Autodesk Inventor part; units mm, degrees
ref_plane "YZ Plane" through (0, 0, 0) normal (1, 0, 0) x (0, 1, 0)
ref_plane "XZ Plane" through (0, 0, 0) normal (0, 1, 0) x (-1, 0, 0)
ref_plane "XY Plane" through (0, 0, 0) normal (0, 0, 1) x (1, 0, 0)
sketch "Sketch1" plane through (0, 0, 0) normal (0, 1, 0) x (-1, 0, 0)
  circle A0 centre (0, 0) radius 17.5
  dimension "d0" = 35
extrude "Extrusion1" add sketch "Sketch1" along normal blind 3
sketch "Sketch2" plane through (0, 3, 0) normal (0, 1, 0) x (1, 0, 0)
  circle A0 centre (0, 0) radius 11
  dimension "d3" = 22
extrude "Extrusion2" add sketch "Sketch2" along normal blind 3
sketch "Sketch3" plane through (0, 0, 0) normal (0, -1, 0) x (1, 0, 0)
  circle A0 centre (0, 0) radius 13.5
  dimension "d6" = 27
extrude "Extrusion3" add sketch "Sketch3" along normal blind 30
fillet "Fillet1" radius 1.5 1 edges at (17.5, 3, 0)
fillet "Fillet2" radius 1.5 1 edges at (-11, 6, 0)
thread "Thread1"
properties part number "Boton" material "ABS Plastic"
Part model, mm, in its own coordinate system. A direction names the side the tool comes from. Give positions to 0.01 mm unless a question says otherwise; leave off trailing zeros. Order: outer loops, then holes, each group sorted by start corner. A loop starts at its lowest first (then second) coordinate and runs counter-clockwise, first axis right, second up. Notation, with made-up numbers: (50, -35) - (57, -35) arc R11 ccw to (57, -25) - close; hole circle Ø10 at (1, 56.5). An arc over 180 degrees is marked (long way). Use one line per item in the form item = value.
Item 1: Slice it at C-C on y = -13. Give the cut face in (x, z), and give its area (3 significant figures).
Solution:
outline = circle Ø27 at (0, 0)
area = 573 mm2
Item 2: Slice it at A-A on z = 0. Give the cut face in (x, y).
Solution:
outline = (-17.5, 0) - (-13.5, 0) - (-13.5, -30) - (13.5, -30) - (13.5, 0) - (17.5, 0) - (17.5, 1.5) arc R1.5 ccw to (16, 3) - (11, 3) - (11, 4.5) arc R1.5 ccw to (9.5, 6) - (-9.5, 6) arc R1.5 ccw to (-11, 4.5) - (-11, 3) - (-16, 3) arc R1.5 ccw to (-17.5, 1.5) - close
Item 3: Probe probe 1 along Y at (x, z) = (-2.5, 12); probe 2 along X at (y, z) = (-26.5, 0.5); probe 3 along X at (y, z) = (2, 7.5). List the from-to ranges inside material, lowest first. Write a range as from..to.
Solution:
probe_1 = -30..3
probe_2 = -13.49..13.49
probe_3 = -15.72..15.72
Item 4: Pin check, flat tips, straight feed: pin 1 Ø8 at (y, z) = (-23, -13) entering from -X; pin 2 Ø5 at (y, z) = (-18.5, -12.5) entering from +X; pin 3 Ø2 at (x, y) = (-13, -7.5) entering from -Z. Stop position of each tip, or through.
Solution:
pin_1 = -10.06
pin_2 = 9.07
pin_3 = -6.18
Item 5: Which spindle directions (+Z, -Z, +X, -X, +Y, -Y) get a long thin tool onto all of the face, cutting with end or side? Do faces 1 (the face through (13.887, 0.74, 10.648)), 2 (the face through (-2.38, 3.74, -10.74)), 3 (the face through (-9, 0, -10.3)). Say none if no direction does.
Solution:
face_1 = +Y, -Y
face_2 = +Y
face_3 = -Y
Item 6: Slice it at B-B on x = 0. Give the cut face in (y, z), and give its area (3 significant figures).
Solution:
outline = (-30, -13.5) - (0, -13.5) - (0, -17.5) - (1.5, -17.5) arc R1.5 ccw to (3, -16) - (3, -11) - (4.5, -11) arc R1.5 ccw to (6, -9.5) - (6, 9.5) arc R1.5 ccw to (4.5, 11) - (3, 11) - (3, 16) arc R1.5 ccw to (1.5, 17.5) - (0, 17.5) - (0, 13.5) - (-30, 13.5) - close
area = 979 mm2
Item 7: Two-plate mould, pull along Y, no slides. Class faces 4 (the face through (-2.93, -14.79, 13.18)), 5 (the face through (0, 6, 0)), 6 (the face through (0, -30, 0)): released by +Y, released by -Y, zero draft, split by the parting line, or undercut.
Solution:
face_4 = zero draft
face_5 = released by +Y
face_6 = released by -Y
